Geometry: see drawing. Coordinates: mm, zero at the bounding-box minimum. A direction names the side the tool comes from. Round coordinates to 2 decimals unless told otherwise and drop trailing zeros. Order: outer loops, then holes, each group sorted by start corner. A loop starts at its lowest first (then second) coordinate and runs counter-clockwise, first axis right, second up. Notation, with made-up numbers: (62, 37.25) -> (84, 37.25) arc R9 ccw to (84, 47.25) -> close; hole circle Ø4 at (61, 52). An arc over 180 degrees is marked (long way). Use a Markdown table: item, result.
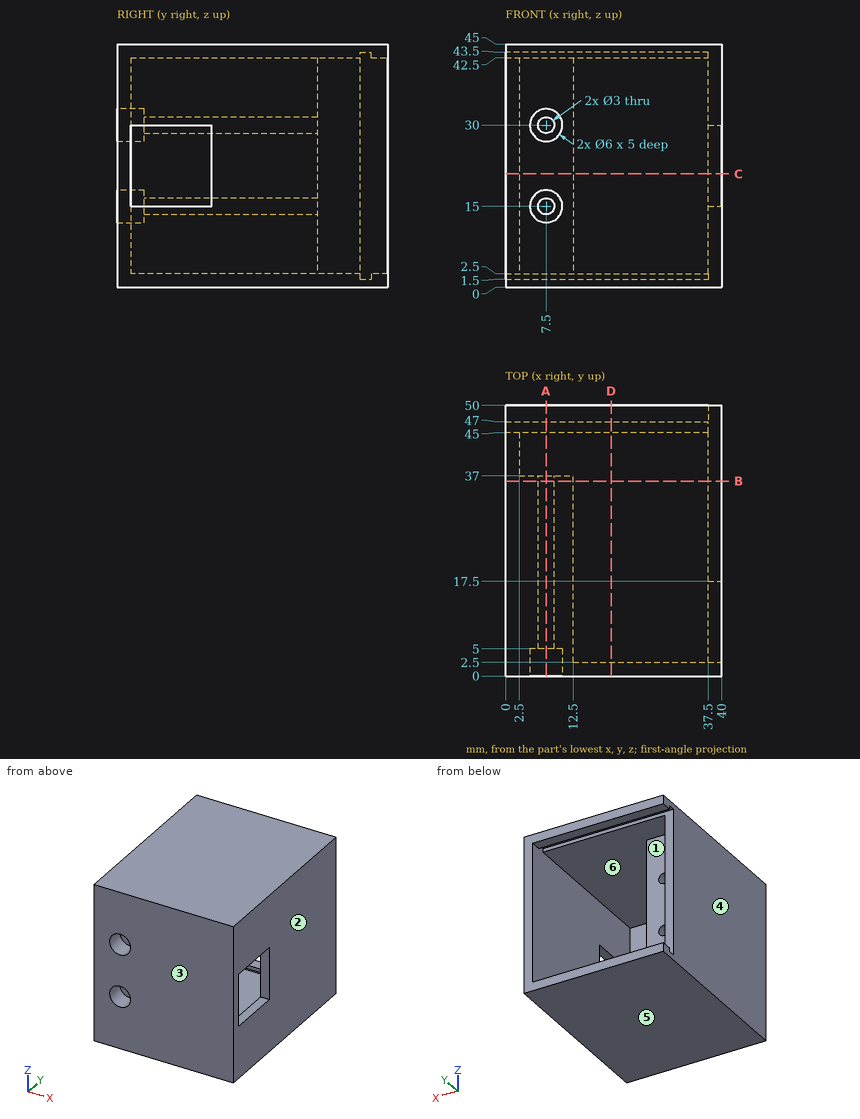
1) Cut plane A-A on x = 7.5. State how many separate pieces and enclosed holes the cut face has, and give its area (3 significant figures).
Answer key:
| item | result |
|---|---|
| separate pieces | 3 |
| enclosed holes | 0 |
| area | 1,470 mm^2 |
2) Cut plane D-D on x = 19.5. Return loops of the section in (y, z).
Answer key:
| item | result |
|---|---|
| outline | (0, 0) -> (50, 0) -> (50, 2.5) -> (47, 2.5) -> (47, 1.5) -> (45, 1.5) -> (45, 2.5) -> (2.5, 2.5) -> (2.5, 42.5) -> (45, 42.5) -> (45, 43.5) -> (47, 43.5) -> (47, 42.5) -> (50, 42.5) -> (50, 45) -> (0, 45) -> close |
3) Set-up query: the marked faces 5 and 6. Return all of +Z, -Z, +X, -X, +Y, -Y with unobstructed straight access to the full face (end or side cutting, diameter ignored); none if empty.
Answer key:
| item | result |
|---|---|
| face 5 | -Z, +X, -X, +Y, -Y |
| face 6 | +Y |
4) Cut plane C-C on z = 21. Return loops of the section in (x, y).
Answer key:
| item | result |
|---|---|
| outline | (0, 0) -> (40, 0) -> (40, 2.5) -> (12.5, 2.5) -> (12.5, 37) -> (2.5, 37) -> (2.5, 45) -> (0, 45) -> close; (37.5, 17.5) -> (40, 17.5) -> (40, 50) -> (37.5, 50) -> close |
5) Contact query for flat-ended pins moving along their axis: P1, Ø2, axis at x = 19.5, z = 25, coming from the +Y side; P2, Ø1.8, axis at x = 7.5, z = 30, coming from the -Y side; P3, Ø3, axis at x = 6.5, z = 15, coming from the -Y side; P4, Ø3, axis at x = 7.5, z = 20.5, coming from the +Y side. Output: stop coordinate, or through.
Answer key:
| item | result |
|---|---|
| P1 | stops at y = 2.5 |
| P2 | passes through |
| P3 | stops at y = 5 |
| P4 | stops at y = 37 |
6) Cut plane B-B on y = 36. Return loops of the section in (x, z).
Answer key:
| item | result |
|---|---|
| outline | (0, 0) -> (40, 0) -> (40, 45) -> (0, 45) -> close; hole circle Ø3 at (7.5, 15); hole circle Ø3 at (7.5, 30); hole (12.5, 2.5) -> (37.5, 2.5) -> (37.5, 42.5) -> (12.5, 42.5) -> close |
7) Draft query along X for the marked faces 1, 2, 3 and 4. Return one class per face: released by +X, released by -X, zero draft, split by the parting line, or undercut.
Answer key:
| item | result |
|---|---|
| face 1 | undercut |
| face 2 | released by +X |
| face 3 | zero draft |
| face 4 | released by -X |
8) Ray query, probe 1 along X at (y, z) = (21, 15); probe 2 along Z at (x, y) = (7, 2); probe 3 along Z at (x, y) = (23, 26.5). Return the intervals inside material, ascending.
Answer key:
| item | result |
|---|---|
| probe 1 | x = 0 to 6, 9 to 12.5, 37.5 to 40 |
| probe 2 | z = 0 to 12.04, 17.96 to 27.04, 32.96 to 45 |
| probe 3 | z = 0 to 2.5, 42.5 to 45 |
